Geometry check sheet. Reference: the model listing, model coordinates, mm. A direction names the side the tool comes from. Coordinates: 2 decimals unless noted, no trailing zeros. Write each loop counter-clockwise with the first axis right and the second up, starting at its lowest first coordinate (ties: lowest second). Pieces come first, ordered by that corner, then holes. Notation, with made-up numbers: (-15.75, -14) -> (-5.75, -14) arc R17 cw to (-5.75, 2) -> close; hole circle Ø3 at (5.5, -35). An arc over 180 degrees is marked (long way). One line per question, with ' | ' between items.
```python
from build123d import *

# Parameters (mm, degrees)
SKETCH1_R           = 11.1125
BOSS_EXTRUDE1_DEPTH = 572.77
BOSS_EXTRUDE2_START = -25.4
SKETCH2_R           = 12.261678201
SKETCH2_R_2         = 11.1125
BOSS_EXTRUDE2_DEPTH = 25.4
SKETCH6_W           = 25.4
SKETCH6_H           = 25.4
BOSS_EXTRUDE3_DEPTH = 25.4
SKETCH7_R           = 6.35
CUT_EXTRUDE1_DEPTH  = 50.8
SKETCH8_R           = 50.8
BOSS_EXTRUDE4_DEPTH = 10.16
FILLET1_R           = 10.16


with BuildPart() as part:
    # Sketch1 → Boss-Extrude1 (new body)
    with BuildSketch(Plane.XY):
        Circle(SKETCH1_R)
    extrude(amount=BOSS_EXTRUDE1_DEPTH)

    # Sketch2 → Boss-Extrude2 (add)
    with BuildSketch(Plane.XY.offset(572.77).offset(BOSS_EXTRUDE2_START)):
        Circle(SKETCH2_R)
        Circle(SKETCH2_R_2, mode=Mode.SUBTRACT)
    extrude(amount=BOSS_EXTRUDE2_DEPTH)

    # Sketch6 → Boss-Extrude3 (add)
    with BuildSketch(Plane.XY.offset(572.77)):
        Rectangle(SKETCH6_W, SKETCH6_H)
    extrude(amount=BOSS_EXTRUDE3_DEPTH)

    # Sketch7 → Cut-Extrude1 (cut)
    with BuildSketch(Plane(origin=(12.7, 0, 0), x_dir=(0, 0, -1), z_dir=(1, 0, 0))):
        with Locations(Location((-588.01, 0, 0), (0, 0, 90))):
            Circle(SKETCH7_R)
    extrude(amount=-CUT_EXTRUDE1_DEPTH, mode=Mode.SUBTRACT)

    # Sketch8 → Boss-Extrude4 (add)
    with BuildSketch(Plane.XY.offset(572.77)):
        Circle(SKETCH8_R)
    extrude(amount=-BOSS_EXTRUDE4_DEPTH)

    # Fillet1
    fillet1_edges = [part.edges().sort_by_distance(p)[0] for p in [
        (0, 12.7, 572.77),
        (0, -12.7, 572.77),
        (0, 12.7, 598.17),
        (0, -12.7, 598.17),
    ]]
    fillet(fillet1_edges, radius=FILLET1_R)


solid = part.part
```
(1) Cross-section at C-C (z = 238). Record the cut outline in (x, y) (1 decimal), plus the area to 3 significant figures.
Answers below:
outline: circle Ø22.2 at (0, 0) | area: 388 mm²
(2) Cross-section at D-D (x = 37). Record the cut outline in (y, z), plus the area to 3 significant figures.
Answers below:
outline: (-34.81, 562.61) -> (34.81, 562.61) -> (34.81, 572.77) -> (-34.81, 572.77) -> close | area: 707 mm²
(3) Cross-section at A-A (x = -2). Record the cut outline in (y, z).
Answers below:
outline: (-50.76, 562.61) -> (-12.1, 562.61) -> (-12.1, 547.37) -> (-10.93, 547.37) -> (-10.93, 0) -> (10.93, 0) -> (10.93, 547.37) -> (12.1, 547.37) -> (12.1, 562.61) -> (50.76, 562.61) -> (50.76, 572.77) -> (22.86, 572.77) arc R10.16 cw to (12.7, 582.93) -> (12.7, 588.01) arc R10.16 ccw to (2.54, 598.17) -> (-2.54, 598.17) arc R10.16 ccw to (-12.7, 588.01) -> (-12.7, 582.93) arc R10.16 cw to (-22.86, 572.77) -> (-50.76, 572.77) -> close; hole circle Ø12.7 at (0, 588.01)
(4) Cross-section at B-B (y = -37.5). Record the cut outline in (x, z), plus the area to 3 significant figures.
Answers below:
outline: (-34.27, 562.61) -> (34.27, 562.61) -> (34.27, 572.77) -> (-34.27, 572.77) -> close | area: 696 mm²
(5) Tool access check on faces 1 (the face through (11, -11, 562.61)), 2 (the face through (0, 0, 0)), 3 (the face through (-12.7, 0, 580)), 4 (the face through (12.7, 0, 580)). Record the directions out of +Z, -Z, +X, -X, +Y, -Y that give a thin tool (end or side, any length) a straight path to the whole face; none if there is none.
Answers below:
face 1: -Z | face 2: -Z, +X, -X, +Y, -Y | face 3: +Z, -X, +Y, -Y | face 4: +Z, +X, +Y, -Y
(6) Depth check by flat-ended pin: P1, Ø4, axis at x = -2.5, z = 584.5, coming from the -Y side; P2, Ø20.5, axis at y = 2.5, z = 588, coming from the +X side; P3, Ø1.5, axis at x = 18.5, y = 10, coming from the +Z side. Enter the tip coordinate at first touch or a pass-through.
Answers below:
P1: stops at y = -12.71 | P2: stops at x = 12.7 | P3: stops at z = 572.77
(7) Material ranges on line 1 (Y direction, x = 0, z = 588); line 2 (Z direction, x = -1.75, y = 0); line 3 (Z direction, x = -24, y = 33), recorded low to high.
Answers below:
line 1: y = -12.7 to -6.35, 6.35 to 12.7 | line 2: z = 0 to 581.66, 594.36 to 598.17 | line 3: z = 562.61 to 572.77
